Work out the finished part from the listing and answer in its coordinate system (mm). A direction names the side the tool comes from. Round coordinates to 2 decimals unless told otherwise and drop trailing zeros. Order: outer loops, then holes, each group sorted by start corner. A loop starts at its lowest first (then second) coordinate and runs counter-clockwise, first axis right, second up. Notation, with made-up numbers: (73.25, 0.5) -> (93.25, 0.5) arc R27 cw to (93.25, 24.5) -> close; hole circle Ø11 at (66.25, 66.25). An arc over 180 degrees is marked (long way). Use one line per item in the form item = value.
```python
from build123d import *

# Parameters (mm, degrees)
BOSS_EXTRUDE1_DEPTH = 3
BOSS_EXTRUDE2_DEPTH = 6
FILLET1_R           = 20
FILLET2_R           = 6
FILLET4_R           = 3
SKETCH4_W           = 77.991272398
SKETCH4_H           = 3
BOSS_EXTRUDE3_DEPTH = 8


with BuildPart() as part:
    # Sketch2 → Boss-Extrude1 (new body)
    with BuildSketch(Plane.XY):
        Polygon((85, 0), (85, 30), (-85, 30), (-85, 0), (-58.995636199, -70), (0, -80), (58.995636199, -70), align=None)
        Polygon((63.885527266, -33), (52.762165892, -62.942485887), (0, -71.885887347), (-52.762165892, -62.942485887), (-63.885527266, -33), align=None, mode=Mode.SUBTRACT)
    extrude(amount=BOSS_EXTRUDE1_DEPTH)

    # Sketch3 → Boss-Extrude2 (add)
    with BuildSketch(Plane.XY.offset(3)):
        Polygon((-74.691839611, -14.825881059), (-55.682056872, -65.99747679), (0, -75.435811633), (55.682056872, -65.99747679), (74.691839611, -14.825881059), (76.82538642, -14.825881059), (57.154758795, -67.776375994), (0, -77.464339796), (-57.154758795, -67.776375994), (-76.82538642, -14.825881059), align=None)
    extrude(amount=BOSS_EXTRUDE2_DEPTH)

    # Fillet1
    fillet1_edges = [part.edges().sort_by_distance(p)[0] for p in [
        (0, -71.885887347, 1.5),
        (0, -75.435811633, 6),
    ]]
    fillet(fillet1_edges, radius=FILLET1_R)

    # Fillet2
    fillet2_edges = [part.edges().sort_by_distance(p)[0] for p in [
        (-52.762165892, -62.942485887, 1.5),
        (52.762165892, -62.942485887, 1.5),
        (55.682056872, -65.99747679, 6),
        (-55.682056872, -65.99747679, 6),
    ]]
    fillet(fillet2_edges, radius=FILLET2_R)

    # Fillet4
    fillet4_edges = [part.edges().sort_by_distance(p)[0] for p in [
        (63.885527266, -33, 1.5),
        (-63.885527266, -33, 1.5),
    ]]
    fillet(fillet4_edges, radius=FILLET4_R)

    # Sketch4 → Boss-Extrude3 (add)
    with BuildSketch(Plane.XY.offset(3)):
        with Locations((0, -31.5)):
            Rectangle(SKETCH4_W, SKETCH4_H)
    extrude(amount=BOSS_EXTRUDE3_DEPTH)


solid = part.part
```
Item 1: Consider line 1 along Z through (x, y) = (23.5, -26); line 2 along Y through (x, z) = (-29.5, 1); line 3 along X through (y, z) = (-59.5, 0.75). Determine where each line is inside the solid, lowest interval first.
Findings:
line_1 = 0 to 3
line_2 = -75 to -66.89, -33 to 30
line_3 = -62.9 to -54.04, 54.04 to 62.9
Item 2: The part is cut by section A-A, the plane z = 5. Give the vertices of the cut face in (x, y).
Findings:
outline = (-76.83, -14.83) -> (-57.15, -67.78) -> (0, -77.46) -> (57.15, -67.78) -> (76.83, -14.83) -> (74.69, -14.83) -> (56.89, -62.75) arc R6 cw to (52.27, -66.58) -> (3.34, -74.87) arc R20 cw to (-3.34, -74.87) -> (-52.27, -66.58) arc R6 cw to (-56.89, -62.75) -> (-74.69, -14.83) -> close; (-39, -33) -> (39, -33) -> (39, -30) -> (-39, -30) -> close
Item 3: The part is cut by section D-D, the plane y = 18. Give the vertices of the cut face in (x, z), and give its area (3 significant figures).
Findings:
outline = (-85, 0) -> (85, 0) -> (85, 3) -> (-85, 3) -> close
area = 510 mm^2
Item 4: The part is cut by section B-B, the plane x = -11. Give the vertices of the cut face in (y, z).
Findings:
outline = (-78.14, 0) -> (-70.02, 0) -> (-70.02, 3) -> (-73.57, 3) -> (-73.57, 9) -> (-75.6, 9) -> (-75.6, 3) -> (-78.14, 3) -> close; (-33, 0) -> (30, 0) -> (30, 3) -> (-30, 3) -> (-30, 11) -> (-33, 11) -> close
Item 5: The part is cut by section C-C, the plane y = -47.5. Give the vertices of the cut face in (x, z).
Findings:
outline = (-67.35, 0) -> (-58.5, 0) -> (-58.5, 3) -> (-62.55, 3) -> (-62.55, 9) -> (-64.69, 9) -> (-64.69, 3) -> (-67.35, 3) -> close; (58.5, 0) -> (67.35, 0) -> (67.35, 3) -> (64.69, 3) -> (64.69, 9) -> (62.55, 9) -> (62.55, 3) -> (58.5, 3) -> close
Item 6: Flat-ended cylindrical pins translate along their axes: P1, Ø5.5, axis at x = 10, z = 6, coming from the -Y side; P2, Ø1.1, axis at x = -76, z = 6, coming from the +Y side; P3, Ø1.5, axis at y = -26, z = 6, coming from the +X side; P4, Ø19, axis at x = -5, y = -50.5, coming from the +Z side. Find the tip coordinate at first contact, or state that the pin passes through.
Findings:
P1 = -76.24
P2 = -14.83
P3 = 72.95
P4 = through
Item 7: Determine the mould class of faces 4 (the cylindrical face through (52.136, -62.255, 1.521)), 5 (the flat face through (-28.177, -72.688, 5.958)), 6 (the flat face through (29.08, -75.07, 1.48)), 7 (the flat face through (-58.117, -48.529, 1.479)) for opening direction X: released by +X, released by -X, zero draft, split by the parting line, or undercut.
Findings:
face_4 = undercut
face_5 = released by -X
face_6 = released by +X
face_7 = undercut
Item 8: For faces 1 (the flat face through (-26.023, -67.475, 1.479)), 2 (the flat face through (27.46, -70.78, 5.96)), 3 (the flat face through (65.665, -39.124, 5.958)), determine the directions among +Z, -Z, +X, -X, +Y, -Y from which every point of the face is accessible in a straight line to the end or side of a thin tool.
Findings:
face_1 = +Z, -Z
face_2 = +Z
face_3 = +Z, +Y
